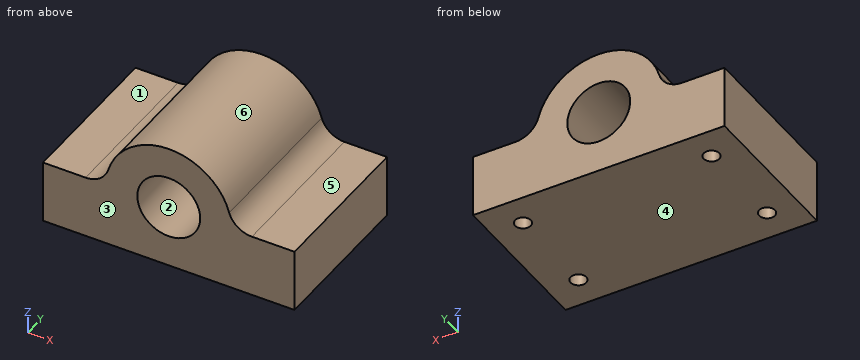
```python
from build123d import *

# Parameters (mm, degrees)
F1_DEPTH = 127
F2_R     = 6.35
F3_DEPTH = 31.75


with BuildPart() as f1:
    # F0 (on Front) → F1 (new body)
    with BuildSketch(Plane.XZ):
        with BuildLine():
            ThreePointArc((67.202083, 0), (55.714501, 3.853357), (48.874242, 13.854545))
            ThreePointArc((48.874242, 13.854545), (0, 50.8), (-48.874242, 13.854545))
            ThreePointArc((-48.874242, 13.854545), (-55.714501, 3.853357), (-67.202083, 0))
            Line((-67.202083, 0), (-101.6, 0))
            Line((-101.6, 0), (-101.6, -50.8))
            Line((-101.6, -50.8), (101.6, -50.8))
            Line((101.6, -50.8), (101.6, 0))
            Line((101.6, 0), (67.202083, 0))
        make_face()
        with BuildLine():
            ThreePointArc((-25.4, 0), (0, 25.4), (25.4, 0))
            ThreePointArc((25.4, 0), (0, -25.4), (-25.4, 0))
        make_face(mode=Mode.SUBTRACT)
    extrude(amount=F1_DEPTH)

    # F2 (on face) → F3 (cut)
    with BuildSketch(Plane(origin=(0, 0, -50.8), x_dir=(1, 0, 0), z_dir=(0, 0, -1))):
        with Locations((-76.2, 101.6)):
            Circle(F2_R)
        with Locations((-76.2, 25.4)):
            Circle(F2_R)
        with Locations((76.2, 25.4)):
            Circle(F2_R)
        with Locations((76.2, 101.6)):
            Circle(F2_R)
    extrude(amount=-F3_DEPTH, mode=Mode.SUBTRACT)


solid = f1.part
```
The listing builds one solid part. Answer for the finished solid, in the listing's coordinates (mm). Face numbers are marked on the shaded views. A direction names the side the tool comes from. Coordinates: 2 decimals unless noted, no trailing zeros. Write each loop counter-clockwise with the first axis right and the second up, starting at its lowest first coordinate (ties: lowest second). Pieces come first, ordered by that corner, then holes. Notation, with made-up numbers: (-25, 30) - (27, 30) arc R21 ccw to (27, 42) - close; hole circle Ø5 at (81.5, 37.5). An arc over 180 degrees is marked (long way). Return JSON: item names as keys, results as strings. Group by question number.
1. Given pin 1 (17 mm diameter, centred on x = -89.5, y = -68.5, fed in from +Z); pin 2 (11.5 mm diameter, centred on x = -76.2, y = -101.6, fed in from -Z), each flat-ended and moving along its own axis, determine where each tip first touches the part or whether it passes through.
2. A cutting plane is placed at A-A, the plane y = -15. Determine the outline of the cut face in (x, z), plus the area to 3 significant figures.
3. A cutting plane is placed at D-D, the plane x = 76.2. Determine the outline of the cut face in (y, z), plus the area to 3 significant figures.
4. A cutting plane is placed at B-B, the plane z = -6. Determine the outline of the cut face in (x, y), plus the area to 3 significant figures.
5. Determine the mould class of the marked faces 1, 2, 3 and 4 for opening direction Z: released by +Z, released by -Z, zero draft, split by the parting line, or undercut.
6. Straight lines are drawn through the part: L1, parallel to Y at x = -76.2, z = -29; L2, parallel to X at y = -101, z = -34; L3, parallel to Z at x = 0, y = -89.5. For each, find the intervals that lie inside material, in ascending order.
7. A cutting plane is placed at C-C, the plane x = 0. Determine the outline of the cut face in (y, z).
8. Which of the six approach directions +Z, -Z, +X, -X, +Y, -Y give full straight-line access (tool end or side, diameter ignored) to the marked faces 5 and 6?
Ans:
{
 "1": {"pin 1": "z = 0", "pin 2": "z = -19.05"},
 "2": {"outline": "(-101.6, -50.8) - (101.6, -50.8) - (101.6, 0) - (67.2, 0) arc R19.05 cw to (48.87, 13.85) arc R50.8 ccw to (-48.87, 13.85) arc R19.05 cw to (-67.2, 0) - (-101.6, 0) - close; hole circle Ø50.8 at (0, 0)", "area": "12,400 mm²"},
 "3": {"outline": "(-127, -50.8) - (-107.95, -50.8) - (-107.95, -19.05) - (-95.25, -19.05) - (-95.25, -50.8) - (-31.75, -50.8) - (-31.75, -19.05) - (-19.05, -19.05) - (-19.05, -50.8) - (0, -50.8) - (0, 0) - (-127, 0) - close", "area": "5,650 mm²"},
 "4": {"outline": "(-101.6, -127) - (-24.68, -127) - (-24.68, 0) - (-101.6, 0) - close; (24.68, -127) - (101.6, -127) - (101.6, 0) - (24.68, 0) - close", "area": "19,500 mm²"},
 "5": {"face 1": "released by +Z", "face 2": "undercut", "face 3": "zero draft", "face 4": "released by -Z"},
 "6": {"L1": "-127 to -107.95, -95.25 to -31.75, -19.05 to 0", "L2": "-101.6 to -82.52, -69.88 to 69.88, 82.52 to 101.6", "L3": "-50.8 to -25.4, 25.4 to 50.8"},
 "7": {"outline": "(-127, -50.8) - (0, -50.8) - (0, -25.4) - (-127, -25.4) - close; (-127, 25.4) - (0, 25.4) - (0, 50.8) - (-127, 50.8) - close"},
 "8": {"face 5": "+Z, +X, +Y, -Y", "face 6": "+Z, +Y, -Y"}
}
